Design review of the part built by this model. Coordinates are the model's own, in mm. Round coordinates to 2 decimals unless told otherwise and drop trailing zeros. Order: outer loops, then holes, each group sorted by start corner. A loop starts at its lowest first (then second) coordinate and runs counter-clockwise, first axis right, second up.
from build123d import *

# Parameters (mm, degrees)
SKETCH1_R           = 10
BOSS_EXTRUDE1_DEPTH = 2
SKETCH2_R           = 3.5
BOSS_EXTRUDE2_DEPTH = 2
SKETCH3_R           = 2.5
CUT_EXTRUDE1_DEPTH  = 15.696938457
SKETCH4_R           = 0.85
CUT_EXTRUDE2_DEPTH  = 15.282856857


with BuildPart() as part:
    # Sketch1 → Boss-Extrude1 (new body)
    with BuildSketch(Plane(origin=(0, 0, 0), x_dir=(1, 0, 0), z_dir=(0, 1, 0))):
        with Locations(Location((0, 0, 0), (0, 0, 270))):
            Circle(SKETCH1_R)
    extrude(amount=BOSS_EXTRUDE1_DEPTH)

    # Sketch2 → Boss-Extrude2 (add)
    with BuildSketch(Plane(origin=(0, 2, 0), x_dir=(1, 0, 0), z_dir=(0, 1, 0))):
        with Locations(Location((0, 0, 0), (0, 0, 270))):
            Circle(SKETCH2_R)
    extrude(amount=BOSS_EXTRUDE2_DEPTH)

    # Sketch3 → Cut-Extrude1 (cut, through all)
    with BuildSketch(Plane(origin=(0, 4, 0), x_dir=(1, 0, 0), z_dir=(0, 1, 0))):
        with Locations(Location((0, 0, 0), (0, 0, 270))):
            Circle(SKETCH3_R)
    extrude(amount=-CUT_EXTRUDE1_DEPTH, mode=Mode.SUBTRACT)

    # Sketch4 → Cut-Extrude2 (cut, through all)
    with BuildSketch(Plane(origin=(0, 2, 0), x_dir=(1, 0, 0), z_dir=(0, 1, 0))):
        with Locations(Location((0, 7.5, 0), (0, 0, 270))):
            Circle(SKETCH4_R)
        with Locations(Location((-7.5, 0, 0), (0, 0, 270))):
            Circle(SKETCH4_R)
        with Locations(Location((7.5, 0, 0), (0, 0, 270))):
            Circle(SKETCH4_R)
        with Locations(Location((0, -7.5, 0), (0, 0, 270))):
            Circle(SKETCH4_R)
    extrude(amount=-CUT_EXTRUDE2_DEPTH, mode=Mode.SUBTRACT)


solid = part.part
1) Take a section at A-A on x = 0. Give the boundary of the cut face in (y, z), plus the area to 3 significant figures.
Results:
outline: (0, -10) - (2, -10) - (2, -8.35) - (0, -8.35) - close; (0, -6.65) - (2, -6.65) - (2, -3.5) - (4, -3.5) - (4, -2.5) - (0, -2.5) - close; (0, 2.5) - (4, 2.5) - (4, 3.5) - (2, 3.5) - (2, 6.65) - (0, 6.65) - close; (0, 8.35) - (2, 8.35) - (2, 10) - (0, 10) - close
area: 27.2 mm2
2) The part is to be moulded in two halves that separate along Z. For faces 1 (the face through (0, 2, 4)), 2 (the face through (0.26, 1.01, -6.69)), 3 (the face through (-3.417, 2.986, -0.759)), say which applies: released by +Z, released by -Z, zero draft, split by the parting line, or undercut.
Results:
face 1: zero draft
face 2: undercut
face 3: split by the parting line
3) Take a section at C-C on y = 1.75. Give the boundary of the cut face in (x, z).
Results:
outline: circle Ø20 at (0, 0); hole circle Ø1.7 at (-7.5, 0); hole circle Ø5 at (0, 0); hole circle Ø1.7 at (0, -7.5); hole circle Ø1.7 at (0, 7.5); hole circle Ø1.7 at (7.5, 0)
4) Take a section at B-B on z = 0. Give the boundary of the cut face in (x, y), plus the area to 3 significant figures.
Results:
outline: (-10, 0) - (-8.35, 0) - (-8.35, 2) - (-10, 2) - close; (-6.65, 0) - (-2.5, 0) - (-2.5, 4) - (-3.5, 4) - (-3.5, 2) - (-6.65, 2) - close; (2.5, 0) - (6.65, 0) - (6.65, 2) - (3.5, 2) - (3.5, 4) - (2.5, 4) - close; (8.35, 0) - (10, 0) - (10, 2) - (8.35, 2) - close
area: 27.2 mm2
5) Clearance check with flat-ended pins moving along their axes: P1, Ø2, axis at x = 0, z = -7.5, coming from the +Y side; P2, Ø1, axis at y = 2, z = 1.5, coming from the +X side. State where each tip first meets the part, or that it passes through.
Results:
P1: stops at y = 2
P2: stops at x = 9.95
6) Take a section at D-D on x = -2.25. Give the boundary of the cut face in (y, z).
Results:
outline: (0, -9.74) - (2, -9.74) - (2, -2.68) - (4, -2.68) - (4, -1.09) - (0, -1.09) - close; (0, 1.09) - (4, 1.09) - (4, 2.68) - (2, 2.68) - (2, 9.74) - (0, 9.74) - close
7) To check wall thickness, follow line 1 along X through (y, z) = (1.75, 0); line 2 along Y through (x, z) = (-3.75, 1.75); line 3 along Z through (x, y) = (0.75, 3.85). State the ranges of each line that lie inside material, in increasing order.
Results:
line 1: x = -10 to -8.35, -6.65 to -2.5, 2.5 to 6.65, 8.35 to 10
line 2: y = 0 to 2
line 3: z = -3.42 to -2.38, 2.38 to 3.42
